Can you work these out from the drawing? Everything is in mm from the part's minimum corner. A direction names the side the tool comes from. Give positions to 0.01 mm unless a question says otherwise; leave off trailing zeros. Loops run counter-clockwise (first coordinate to the right, second up) from the corner with the lowest first, then second, coordinate; pieces in that order, holes last. Notation, with made-up numbers: (48, 1) - (86, 1) arc R25 cw to (86, 36) - close; hole circle Ø3 at (59.5, 3.5). An arc over 180 degrees is marked (long way). Answer in a Markdown table with one row per item.
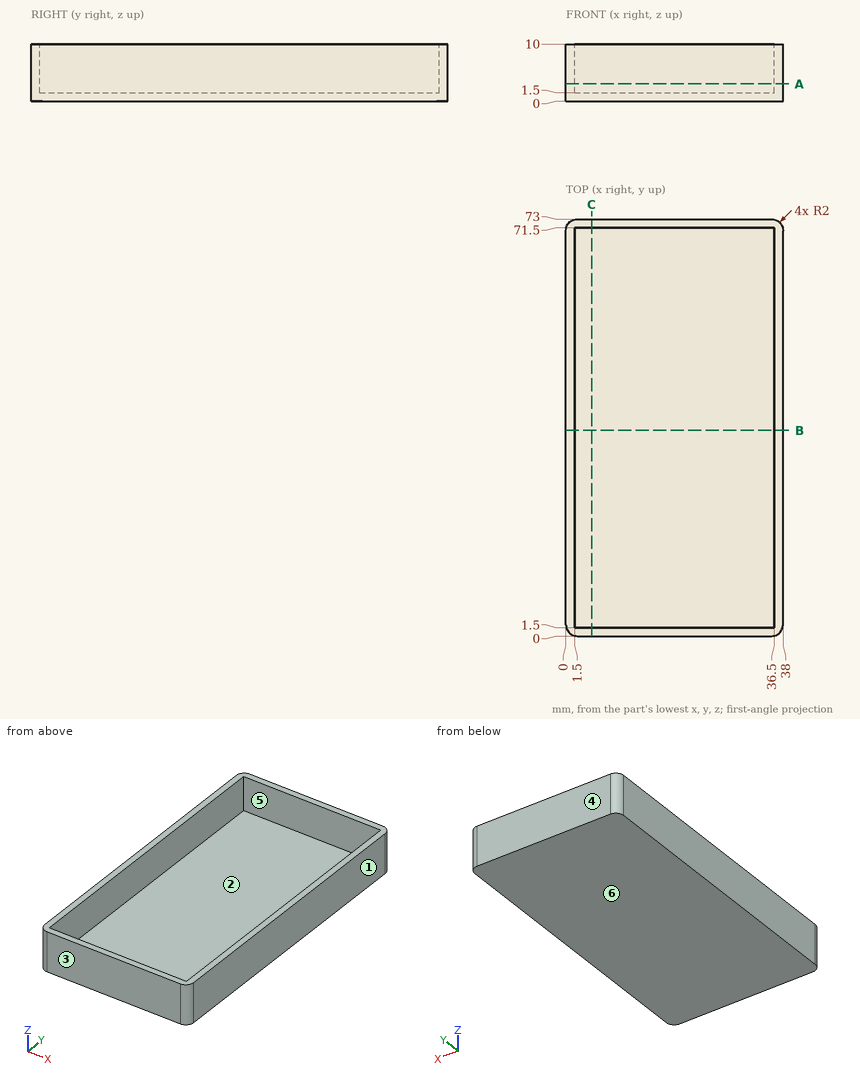
Q1. Imagine slicing it at C-C, the plane x = 4.5. Write out the boundary of the cut face in (y, z), and give its area (3 significant figures).
Checked values:
| item | result |
|---|---|
| outline | (0, 0) - (73, 0) - (73, 10) - (71.5, 10) - (71.5, 1.5) - (1.5, 1.5) - (1.5, 10) - (0, 10) - close |
| area | 135 mm² |
Q2. On a 3-axis mill with a long thin cutter (end or side, diameter ignored), from which of +Z, -Z, +X, -X, +Y, -Y can I reach the whole of each face in a straight line? I mean the marked faces 1 and 2. Say none if no direction works.
Checked values:
| item | result |
|---|---|
| face 1 | +Z, -Z, +X, +Y, -Y |
| face 2 | +Z |
Q3. For pin 1 (4 mm diameter, centred on x = 15.5, y = 58.5, fed in from +Z), with a flat end and sliding along its axis, tell me the tip position at first contact or that it passes through.
Checked values:
| item | result |
|---|---|
| pin 1 | stops at z = 1.5 |
Q4. Imagine slicing it at B-B, the plane y = 36. Write out the boundary of the cut face in (x, z), and give its area (3 significant figures).
Checked values:
| item | result |
|---|---|
| outline | (0, 0) - (38, 0) - (38, 10) - (36.5, 10) - (36.5, 1.5) - (1.5, 1.5) - (1.5, 10) - (0, 10) - close |
| area | 82.5 mm² |
Q5. If I drill on line 1 (X direction, y = 29.5, z = 5.75); line 2 (Y direction, x = 11.5, z = 4.25); line 3 (Z direction, x = 14, y = 65.5), over which ranges is the centre line in solid material (lowest first)? Write a range as [from, to].
Checked values:
| item | result |
|---|---|
| line 1 | x = [0, 1.5], [36.5, 38] |
| line 2 | y = [0, 1.5], [71.5, 73] |
| line 3 | z = [0, 1.5] |
Q6. Imagine slicing it at A-A, the plane z = 3. Write out the boundary of the cut face in (x, y), and give its area (3 significant figures).
Checked values:
| item | result |
|---|---|
| outline | (0, 2) arc R2 ccw to (2, 0) - (36, 0) arc R2 ccw to (38, 2) - (38, 71) arc R2 ccw to (36, 73) - (2, 73) arc R2 ccw to (0, 71) - close; hole (1.5, 1.5) - (36.5, 1.5) - (36.5, 71.5) - (1.5, 71.5) - close |
| area | 321 mm² |
Q7. If we mould it in two halves opening along Y, with no side actions, what happens to the marked faces 3, 4, 5 and 6? For each: released by +Y, released by -Y, zero draft, split by the parting line, or undercut.
Checked values:
| item | result |
|---|---|
| face 3 | released by -Y |
| face 4 | released by +Y |
| face 5 | undercut |
| face 6 | zero draft |
